Geometry check sheet. Reference: the model listing, model coordinates, mm. A direction names the side the tool comes from. Round coordinates to 2 decimals unless told otherwise and drop trailing zeros. Order: outer loops, then holes, each group sorted by start corner. A loop starts at its lowest first (then second) coordinate and runs counter-clockwise, first axis right, second up.
(1) Sectioned sample at D-D (x = 18). Record the boundary of the cut face in (y, z), plus the area to 3 significant figures.
(2) Sectioned sample at C-C (y = 72). Record the boundary of the cut face in (x, z), plus the area to 3 significant figures.
(3) Sectioned sample at A-A (x = -12). Record the boundary of the cut face in (y, z).
(4) Go/stop test with flat-tipped pins: pin 1 (12 mm diameter, centred on x = 192.5, y = 73.5, fed in from +Z); pin 2 (12 mm diameter, centred on x = 152.5, z = 19, fed in from -Y); pin 3 (7 mm diameter, centred on x = 85, z = 36, fed in from +Y). Record where each tip stops, or that it passes through.
(5) Set-up check for faces 1 (the face through (153, 20.208, 64)), 2 (the face through (119.483, 63.168, 48.215)), 3 (the face through (117, 45, 45.75)), 4 (the face through (202, 62, 68.25)), 5 (the face through (202, 62, 28.25)): record each of +Z, -Z, +X, -X, +Y, -Y from which the full face is reachable in a straight line by a thin tool's end or side.
(6) Material ranges on line 1 along X through (y, z) = (-11.5, 68.5); line 2 along X through (y, z) = (49.5, 39); line 3 along Z through (x, y) = (211, 29), recorded low to high.
(7) Release check for a two-part mould opening along Y. For faces 6 (the face through (212.489, 62, 48)), 7 (the face through (125.9, -5.56, 48.72)), 8 (the face through (140.184, 19.297, 64.278)), 9 (the face through (63.494, -15.572, 48.825)) record: +Y half, -Y half, draft (parallel to the pull), parting line (faces both ways), or undercut.
(8) Sectioned sample at B-B (y = 37.5). Record the boundary of the cut face in (x, z).
from build123d import *

# Parameters (mm, degrees)
SKETCH1_W           = 257
SKETCH1_H           = 133.5
BOSS_EXTRUDE1_DEPTH = 96.5
SKETCH2_W           = 113
SKETCH2_H           = 45.5
SKETCH2_W_2         = 80
SKETCH2_H_2         = 40
CUT_EXTRUDE1_DEPTH  = 96.5
CUT_EXTRUDE2_DEPTH  = 88
SKETCH6_W           = 20
SKETCH6_H           = 28.25
CUT_EXTRUDE3_DEPTH  = 93.5
SKETCH7_W           = 124
SKETCH7_H           = 28.25
CUT_EXTRUDE4_DEPTH  = 73.5
SKETCH8_W           = 104
SKETCH8_H           = 17.5
CUT_EXTRUDE5_DEPTH  = 73.5
SKETCH9_W           = 25
SKETCH9_H           = 45.75
CUT_EXTRUDE6_DEPTH  = 68
SKETCH11_W          = 84
SKETCH11_H          = 45.75
CUT_EXTRUDE7_DEPTH  = 14
SKETCH12_W          = 84
SKETCH12_H          = 45.75
CUT_EXTRUDE8_DEPTH  = 14
CUT_EXTRUDE10_DEPTH = 45.75
CUT_EXTRUDE11_DEPTH = 96.5
CUT_EXTRUDE12_DEPTH = 45.75
CUT_EXTRUDE13_DEPTH = 5
SKETCH18_R          = 5
CUT_EXTRUDE14_DEPTH = 96.5
SKETCH19_W          = 20
SKETCH19_H          = 20
CUT_EXTRUDE15_DEPTH = 93.5
CUT_EXTRUDE42_DEPTH = 88
CUT_EXTRUDE53_DEPTH = 20
CUT_EXTRUDE61_DEPTH = 50.68
CUT_EXTRUDE62_DEPTH = 88
CUT_EXTRUDE63_DEPTH = 88
CUT_EXTRUDE64_DEPTH = 88
FILLET2_R           = 10
FILLET3_R           = 10
FILLET4_R           = 10
FILLET5_R           = 10
FILLET6_R           = 10
FILLET7_R           = 10
FILLET8_R           = 10
FILLET9_R           = 10
FILLET10_R          = 10
FILLET11_R          = 10
FILLET12_R          = 10
FILLET13_R          = 10


with BuildPart() as part:
    # Sketch1 → Boss-Extrude1 (new body)
    with BuildSketch(Plane.XY):
        with Locations((93.989304803, 40.957796221)):
            Rectangle(SKETCH1_W, SKETCH1_H)
    extrude(amount=BOSS_EXTRUDE1_DEPTH)

    # Sketch2 → Cut-Extrude1 (cut)
    with BuildSketch(Plane.XY.offset(96.5)):
        with Locations((21.989304803, 84.957796221)):
            Rectangle(SKETCH2_W, SKETCH2_H)
        with Locations((182.489304803, -5.792203779)):
            Rectangle(SKETCH2_W_2, SKETCH2_H_2)
    extrude(amount=-CUT_EXTRUDE1_DEPTH, mode=Mode.SUBTRACT)

    # Sketch4 → Cut-Extrude2 (cut)
    with BuildSketch(Plane(origin=(0, 62.207796221, 0), x_dir=(1, 0, 0), z_dir=(0, 1, 0))):
        Polygon((-24.510695197, -10), (-24.510695197, -48.25), (-24.510695197, -86.5), (43.489304803, -86.5), (43.489304803, -48.25), (43.489304803, -10), align=None)
    extrude(amount=-CUT_EXTRUDE2_DEPTH, mode=Mode.SUBTRACT)

    # Sketch6 → Cut-Extrude3 (cut)
    with BuildSketch(Plane(origin=(0, 107.707796221, 0), x_dir=(1, 0, 0), z_dir=(0, 1, 0))):
        with Locations((212.489304803, -14.125)):
            Rectangle(SKETCH6_W, SKETCH6_H)
        with Locations((212.489304803, -82.375)):
            Rectangle(SKETCH6_W, SKETCH6_H)
    extrude(amount=-CUT_EXTRUDE3_DEPTH, mode=Mode.SUBTRACT)

    # Sketch7 → Cut-Extrude4 (cut)
    with BuildSketch(Plane(origin=(0, 107.707796221, 0), x_dir=(1, 0, 0), z_dir=(0, 1, 0))):
        with Locations((140.489304803, -14.125)):
            Rectangle(SKETCH7_W, SKETCH7_H)
        with Locations((140.489304803, -82.375)):
            Rectangle(SKETCH7_W, SKETCH7_H)
    extrude(amount=-CUT_EXTRUDE4_DEPTH, mode=Mode.SUBTRACT)

    # Sketch8 → Cut-Extrude5 (cut)
    with BuildSketch(Plane(origin=(0, 107.707796221, 0), x_dir=(1, 0, 0), z_dir=(0, 1, 0))):
        with Locations((130.489304803, -37)):
            Rectangle(SKETCH8_W, SKETCH8_H)
        with Locations((130.489304803, -59.5)):
            Rectangle(SKETCH8_W, SKETCH8_H)
    extrude(amount=-CUT_EXTRUDE5_DEPTH, mode=Mode.SUBTRACT)

    # Sketch9 → Cut-Extrude6 (cut)
    with BuildSketch(Plane(origin=(0, 62.207796221, 0), x_dir=(1, 0, 0), z_dir=(0, 1, 0))):
        with Locations((65.989304803, -73.625)):
            Rectangle(SKETCH9_W, SKETCH9_H)
        with Locations((65.989304803, -22.875)):
            Rectangle(SKETCH9_W, SKETCH9_H)
    extrude(amount=-CUT_EXTRUDE6_DEPTH, mode=Mode.SUBTRACT)

    # Sketch11 → Cut-Extrude7 (cut)
    with BuildSketch(Plane(origin=(0, 34.207796221, 0), x_dir=(1, 0, 0), z_dir=(0, 1, 0))):
        with Locations((120.489304803, -73.625)):
            Rectangle(SKETCH11_W, SKETCH11_H)
    extrude(amount=-CUT_EXTRUDE7_DEPTH, mode=Mode.SUBTRACT)

    # Sketch12 → Cut-Extrude8 (cut)
    with BuildSketch(Plane(origin=(0, 34.207796221, 0), x_dir=(1, 0, 0), z_dir=(0, 1, 0))):
        with Locations((120.489304803, -22.875)):
            Rectangle(SKETCH12_W, SKETCH12_H)
    extrude(amount=-CUT_EXTRUDE8_DEPTH, mode=Mode.SUBTRACT)

    # Sketch13 → Cut-Extrude10 (cut)
    with BuildSketch(Plane.XY.offset(96.5)):
        Polygon((139.691458854, 20.207796221), (106.127473607, -19.792203779), (78.489304803, -19.792203779), (78.489304803, 20.207796221), align=None)
    extrude(amount=-CUT_EXTRUDE10_DEPTH, mode=Mode.SUBTRACT)

    # Sketch15 → Cut-Extrude11 (cut)
    with BuildSketch(Plane.XY.offset(96.5)):
        Polygon((142.489304803, 14.207796221), (108.925319556, -25.792203779), (142.489304803, -25.792203779), align=None)
    extrude(amount=-CUT_EXTRUDE11_DEPTH, mode=Mode.SUBTRACT)

    # Sketch16 → Cut-Extrude12 (cut)
    with BuildSketch(Plane(origin=(0, 0, 0), x_dir=(-1, 0, 0), z_dir=(0, 0, -1))):
        Polygon((-78.489304803, -19.792203779), (-106.127473607, -19.792203779), (-139.691458854, 20.207796221), (-78.489304803, 20.207796221), align=None)
    extrude(amount=-CUT_EXTRUDE12_DEPTH, mode=Mode.SUBTRACT)

    # Sketch17 → Cut-Extrude13 (cut)
    with BuildSketch(Plane.XY.offset(50.75)):
        Polygon((78.489304803, 62.207796221), (119.862118509, 62.207796221), (158.148215693, 107.707796221), (78.489304803, 107.707796221), align=None)
    extrude(amount=-CUT_EXTRUDE13_DEPTH, mode=Mode.SUBTRACT)

    # Sketch18 → Cut-Extrude14 (cut)
    with BuildSketch(Plane.XY.offset(96.5)):
        with Locations((172.489304803, 24.207796221)):
            Circle(SKETCH18_R)
        with Locations((68.489304803, -15.792203779)):
            Circle(SKETCH18_R)
    extrude(amount=-CUT_EXTRUDE14_DEPTH, mode=Mode.SUBTRACT)

    # Sketch19 → Cut-Extrude15 (cut)
    with BuildSketch(Plane(origin=(0, 107.707796221, 0), x_dir=(1, 0, 0), z_dir=(0, 1, 0))):
        with Locations((202.489304803, -48.25)):
            Rectangle(SKETCH19_W, SKETCH19_H)
    extrude(amount=-CUT_EXTRUDE15_DEPTH, mode=Mode.SUBTRACT)

    # Sketch51 → Cut-Extrude42 (cut)
    with BuildSketch(Plane(origin=(0, 62.207796221, 0), x_dir=(1, 0, 0), z_dir=(0, 1, 0))):
        Polygon((15.489304803, -96.5), (53.489304803, -96.5), (53.489304803, -90.759358289), align=None)
    extrude(amount=-CUT_EXTRUDE42_DEPTH, mode=Mode.SUBTRACT)

    # Sketch62 → Cut-Extrude53 (cut)
    with BuildSketch(Plane.XZ.offset(-14.207796221)):
        Polygon((142.489304803, 96.5), (202.489304803, 96.5), (202.489304803, 68.25), (142.489304803, 77.314171123), align=None)
    extrude(amount=-CUT_EXTRUDE53_DEPTH, mode=Mode.SUBTRACT)

    # Sketch75 → Cut-Extrude61 (cut)
    with BuildSketch(Plane.XZ.offset(25.792203779)):
        Polygon((142.489304803, 77.314171123), (53.489304803, 90.759358289), (53.489304803, 96.5), (142.489304803, 96.5), align=None)
    extrude(amount=-CUT_EXTRUDE61_DEPTH, mode=Mode.SUBTRACT)

    # Sketch79 → Cut-Extrude62 (cut)
    with BuildSketch(Plane(origin=(0, 62.207796221, 0), x_dir=(1, 0, 0), z_dir=(0, 1, 0))):
        Polygon((15.489304803, 0), (53.489304803, 0), (53.489304803, -5.740641711), align=None)
    extrude(amount=-CUT_EXTRUDE62_DEPTH, mode=Mode.SUBTRACT)

    # Sketch80 → Cut-Extrude63 (cut)
    with BuildSketch(Plane.XZ.offset(25.792203779)):
        Polygon((53.489304803, 5.740641711), (53.489304803, 0), (142.489304803, 0), (142.489304803, 19.185828877), align=None)
    extrude(amount=-CUT_EXTRUDE63_DEPTH, mode=Mode.SUBTRACT)

    # Sketch81 → Cut-Extrude64 (cut)
    with BuildSketch(Plane.XZ.offset(-14.207796221)):
        Polygon((142.489304803, 19.185828877), (202.489304803, 28.25), (202.489304803, 0), (142.489304803, 0), align=None)
    extrude(amount=-CUT_EXTRUDE64_DEPTH, mode=Mode.SUBTRACT)

    # Fillet2
    fillet2_edges = [part.edges().sort_by_distance(p)[0] for p in [
        (162.489304803, 34.207796221, 62.521390374),
    ]]
    fillet(fillet2_edges, radius=FILLET2_R)

    # Fillet3
    fillet3_edges = [part.edges().sort_by_distance(p)[0] for p in [
        (162.489304803, 34.207796221, 33.978609626),
    ]]
    fillet(fillet3_edges, radius=FILLET3_R)

    # Fillet4
    fillet4_edges = [part.edges().sort_by_distance(p)[0] for p in [
        (139.691458854, 20.207796221, 32.256579818),
    ]]
    fillet(fillet4_edges, radius=FILLET4_R)

    # Fillet5
    fillet5_edges = [part.edges().sort_by_distance(p)[0] for p in [
        (139.691458854, 20.207796221, 64.243420182),
    ]]
    fillet(fillet5_edges, radius=FILLET5_R)

    # Fillet6
    fillet6_edges = [part.edges().sort_by_distance(p)[0] for p in [
        (106.127473607, -19.792203779, 66.778667731),
    ]]
    fillet(fillet6_edges, radius=FILLET6_R)

    # Fillet7
    fillet7_edges = [part.edges().sort_by_distance(p)[0] for p in [
        (106.127473607, -19.792203779, 29.721332269),
    ]]
    fillet(fillet7_edges, radius=FILLET7_R)

    # Fillet8
    fillet8_edges = [part.edges().sort_by_distance(p)[0] for p in [
        (78.489304803, -5.792203779, 68.86631016),
    ]]
    fillet(fillet8_edges, radius=FILLET8_R)

    # Fillet9
    fillet9_edges = [part.edges().sort_by_distance(p)[0] for p in [
        (78.489304803, -5.792203779, 27.63368984),
    ]]
    fillet(fillet9_edges, radius=FILLET9_R)

    # Fillet10
    fillet10_edges = [part.edges().sort_by_distance(p)[0] for p in [
        (158.148215693, 107.707796221, 48.25),
    ]]
    fillet(fillet10_edges, radius=FILLET10_R)

    # Fillet11
    fillet11_edges = [part.edges().sort_by_distance(p)[0] for p in [
        (119.862118509, 62.207796221, 48.25),
    ]]
    fillet(fillet11_edges, radius=FILLET11_R)

    # Fillet12
    fillet12_edges = [part.edges().sort_by_distance(p)[0] for p in [
        (142.489304803, 14.207796221, 48.25),
    ]]
    fillet(fillet12_edges, radius=FILLET12_R)

    # Fillet13
    fillet13_edges = [part.edges().sort_by_distance(p)[0] for p in [
        (108.925319556, -25.792203779, 48.25),
    ]]
    fillet(fillet13_edges, radius=FILLET13_R)


solid = part.part
Answer below:
1. outline: (-25.79, 0.38) - (62.21, 0.38) - (62.21, 10) - (-25.79, 10) - close; (-25.79, 86.5) - (62.21, 86.5) - (62.21, 96.12) - (-25.79, 96.12) - close
1. area: 1,690 mm2
2. outline: (128.1, 45.75) - (182.49, 45.75) - (182.49, 28.25) - (222.49, 28.25) - (222.49, 68.25) - (182.49, 68.25) - (182.49, 50.75) - (128.1, 50.75) - close; hole (192.49, 38.25) - (212.49, 38.25) - (212.49, 58.25) - (192.49, 58.25) - close
2. area: 1,470 mm2
3. outline: (-25.79, 0) - (62.21, 0) - (62.21, 10) - (-25.79, 10) - close; (-25.79, 86.5) - (62.21, 86.5) - (62.21, 96.5) - (-25.79, 96.5) - close
4. pin 1: stops at z = 68.25
4. pin 2: stops at y = 14.19
4. pin 3: stops at y = -19.79
5. face 1: +Z, +Y
5. face 2: +Z, -Z, -X, +Y
5. face 3: -Z, +Y
5. face 4: +Z, +X, +Y
5. face 5: -Z, +X, +Y
6. line 1: x = -34.51 to -24.51, 43.49 to 65.92, 71.05 to 77.52, 113.09 to 120.92
6. line 2: x = -34.51 to -24.51, 43.49 to 53.49, 182.49 to 192.49, 212.49 to 222.49
6. line 3: z = 28.25 to 38.25, 58.25 to 68.25
7. face 6: draft
7. face 7: -Y half
7. face 8: +Y half
7. face 9: undercut
8. outline: (-34.51, 0) - (15.49, 0) - (53.49, 5.74) - (53.49, 45.75) - (182.49, 45.75) - (182.49, 28.25) - (222.49, 28.25) - (222.49, 68.25) - (182.49, 68.25) - (182.49, 50.75) - (53.49, 50.75) - (53.49, 90.76) - (15.49, 96.5) - (-34.51, 96.5) - close; hole (-24.51, 10) - (43.49, 10) - (43.49, 86.5) - (-24.51, 86.5) - close; hole (192.49, 38.25) - (212.49, 38.25) - (212.49, 58.25) - (192.49, 58.25) - close
